Check sheet for the modelled part. Datum: model origin and axes. Units: mm. Round coordinates to 2 decimals unless told otherwise and drop trailing zeros. Order: outer loops, then holes, each group sorted by start corner. A loop starts at its lowest first (then second) coordinate and runs counter-clockwise, first axis right, second up. Notation, with made-up numbers: (12.25, -14) -> (60.25, -14) arc R24 cw to (60.25, 11) -> close; hole circle Ø4 at (-16, 85). An arc over 180 degrees is marked (long way). Use CSV: the item, a comma, the result in double quotes.
```python
from build123d import *

# Parameters (mm, degrees)
F0_W     = 10
F0_H     = 104
F1_DEPTH = 247.5
F3_D     = 9
F3_DEPTH = 18
F3_TIP   = 2.7038727856
F5_D     = 9
F5_DEPTH = 18
F5_TIP   = 2.7038727856


with BuildPart() as f1:
    # F0 (on Right) → F1 (new body, symmetric)
    with BuildSketch(Plane.YZ):
        Rectangle(F0_W, F0_H)
    extrude(amount=F1_DEPTH, both=True)

    # F3
    with Locations(Plane.XZ.offset(5)):
        with Locations((-192.5, 28.7598677054), (-237.5, -26.2401322946), (237.5, 28.7598677054), (192.5, -26.2401322946)):
            Hole(F3_D / 2, depth=F3_DEPTH)
            with Locations((0, 0, -(F3_DEPTH + F3_TIP / 2))):  # 118° drill point
                Cone(0, F3_D / 2, F3_TIP, mode=Mode.SUBTRACT)

    # F5
    with Locations(Plane(origin=(0, 5, 0), x_dir=(-1, 0, 0), z_dir=(0, 1, 0))):
        with Locations((-20, 20), (20, 20), (-20, -20), (20, -20), (91, 30), (91, -30), (-91, -30), (-91, 30)):
            Hole(F5_D / 2, depth=F5_DEPTH)
            with Locations((0, 0, -(F5_DEPTH + F5_TIP / 2))):  # 118° drill point
                Cone(0, F5_D / 2, F5_TIP, mode=Mode.SUBTRACT)


solid = f1.part
```
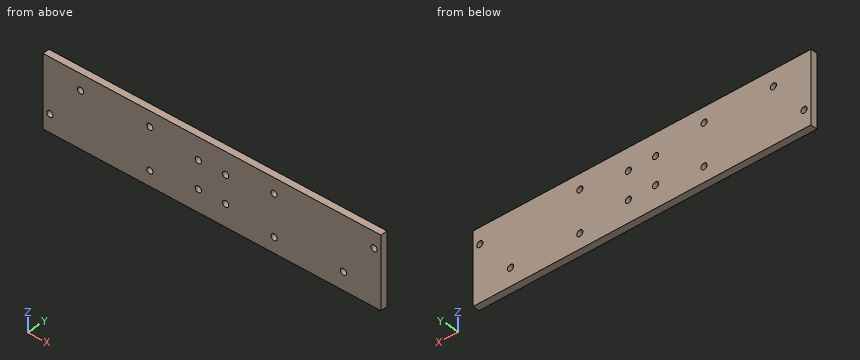
Q1. Scan lines: L1, parallel to Z at x = 20, y = 2.75; L2, parallel to X at y = 4.5, z = -19; L3, parallel to X at y = 3, z = 24. Record each from-to range of solid material in increasing order.
Result sheet:
L1,"z = -52 to -24.5, -15.5 to 15.5, 24.5 to 52"
L2,"x = -247.5 to -24.39, -15.61 to 15.61, 24.39 to 247.5"
L3,"x = -247.5 to -22.06, -17.94 to 17.94, 22.06 to 247.5"
Q2. Go/stop test with a flat-tipped pin: pin 1 (5.5 mm diameter, centred on x = 192.5, z = -26.24, fed in from -Y). Record where the tip stops, or that it passes through.
Result sheet:
pin 1,"passes through"
Q3. Sectioned sample at A-A, the plane x = -237.5. Enter the section's corners in (y, z).
Result sheet:
outline,"(-5, -52) -> (5, -52) -> (5, -30.74) -> (-5, -30.74) -> close; (-5, -21.74) -> (5, -21.74) -> (5, 52) -> (-5, 52) -> close"
Q4. Sectioned sample at B-B, the plane x = 20. Enter the section's corners in (y, z), then the cut area to 3 significant figures.
Result sheet:
outline,"(-5, -52) -> (5, -52) -> (5, -24.5) -> (-5, -24.5) -> close; (-5, -15.5) -> (5, -15.5) -> (5, 15.5) -> (-5, 15.5) -> close; (-5, 24.5) -> (5, 24.5) -> (5, 52) -> (-5, 52) -> close"
area,"860 mm^2"
